Answer from the drawing. Dimensions are ordinates in mm from the lowest x, y and z of the part. A direction names the side the tool comes from. Coordinates: 2 decimals unless noted, no trailing zeros. Write each loop counter-clockwise with the first axis right and the second up, starting at its lowest first coordinate (ties: lowest second). Pieces come first, ordered by that corner, then holes. Notation, with made-up numbers: (-3, 50.25) - (48, 50.25) arc R35 cw to (48, 87.25) - close; hole circle Ø1 at (67, 12.5). An arc over 180 degrees is marked (long way). Use a Markdown table: item, result.
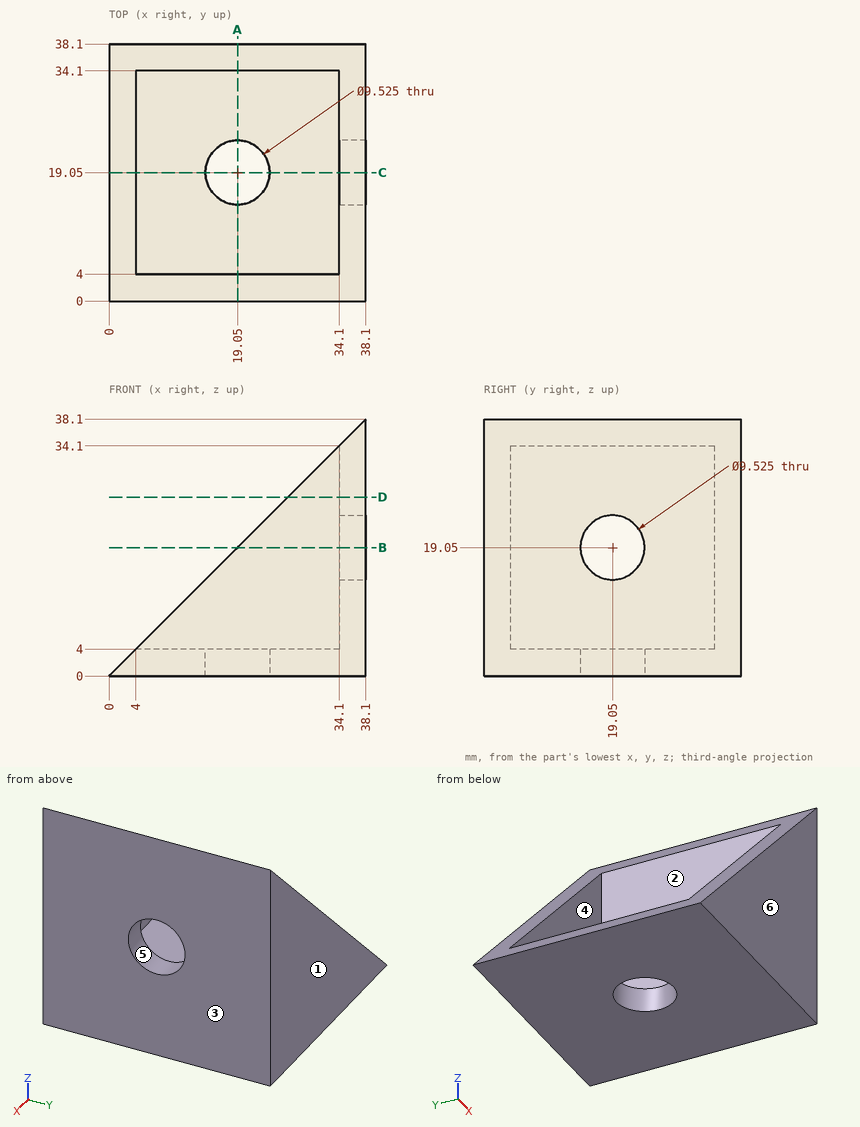
(1) Straight lines are drawn through the part: L1, parallel to Y at x = 19, z = 2; L2, parallel to Y at x = 14, z = 10; L3, parallel to X at y = 9, z = 18. For each, find the intervals that lie inside material, in ascending order.
Report:
| item | result |
|---|---|
| L1 | y = 0 to 14.29, 23.81 to 38.1 |
| L2 | y = 0 to 4, 34.1 to 38.1 |
| L3 | x = 34.1 to 38.1 |
(2) A cutting plane is placed at B-B, the plane z = 19.05. Write down the section's boundary in (x, y), and give its area (3 significant figures).
Report:
| item | result |
|---|---|
| outline | (19.05, 0) - (38.1, 0) - (38.1, 14.29) - (34.1, 14.29) - (34.1, 4) - (19.05, 4) - close; (19.05, 34.1) - (34.1, 34.1) - (34.1, 23.81) - (38.1, 23.81) - (38.1, 38.1) - (19.05, 38.1) - close |
| area | 235 mm² |
(3) A cutting plane is placed at D-D, the plane z = 26.5. Write down the section's boundary in (x, y), and give its area (3 significant figures).
Report:
| item | result |
|---|---|
| outline | (26.5, 0) - (38.1, 0) - (38.1, 38.1) - (26.5, 38.1) - (26.5, 34.1) - (34.1, 34.1) - (34.1, 4) - (26.5, 4) - close |
| area | 213 mm² |
(4) A cutting plane is placed at C-C, the plane y = 19.05. Write down the section's boundary in (x, z).
Report:
| item | result |
|---|---|
| outline | (0, 0) - (14.29, 0) - (14.29, 4) - (4, 4) - close; (23.81, 0) - (38.1, 0) - (38.1, 14.29) - (34.1, 14.29) - (34.1, 4) - (23.81, 4) - close; (34.1, 23.81) - (38.1, 23.81) - (38.1, 38.1) - (34.1, 34.1) - close |
(5) Each of these flat-tipped pins is pushed along its axis until it touches: P1, Ø12.5, axis at y = 19.05, z = 19.05, coming from the -X side; P2, Ø5, axis at y = 32, z = 4, coming from the -X side. Where does it stop, or does it pass through?
Report:
| item | result |
|---|---|
| P1 | stops at x = 34.1 |
| P2 | stops at x = 1.5 |
(6) For the marked faces 1 and 2, determine the directions among +Z, -Z, +X, -X, +Y, -Y from which every point of the face is accessible in a straight line to the end or side of a thin tool.
Report:
| item | result |
|---|---|
| face 1 | +Z, -Z, +X, -X, +Y |
| face 2 | +Z, -X |
(7) A cutting plane is placed at A-A, the plane x = 19.05. Write down the section's boundary in (y, z).
Report:
| item | result |
|---|---|
| outline | (0, 0) - (14.29, 0) - (14.29, 4) - (4, 4) - (4, 19.05) - (0, 19.05) - close; (23.81, 0) - (38.1, 0) - (38.1, 19.05) - (34.1, 19.05) - (34.1, 4) - (23.81, 4) - close |
(8) The mould has two halves that part along Y. Classify the marked faces 3, 4, 5 and 6: pulls with the +Y half, pulls with the -Y half, needs draft (parallel to the pull), parting line crosses it, or undercut.
Report:
| item | result |
|---|---|
| face 3 | needs draft |
| face 4 | undercut |
| face 5 | undercut |
| face 6 | pulls with the -Y half |
